Verification items for the finished model (mm, model axes). Coordinates: 2 decimals unless noted, no trailing zeros. Order: outer loops, then holes, each group sorted by start corner. A loop starts at its lowest first (then second) coordinate and runs counter-clockwise, first axis right, second up. Notation, with made-up numbers: M 29.5,30 L 75.5,30 A12 ccw 75.5,48 Z; hole C 40.25,20.5 d1. An arc over 180 degrees is marked long. Answer as a JSON object with one key per item and string values. Group by question number.
(1) Material ranges on line 1 (Z direction, x = -75, y = 0.7); line 2 (Z direction, x = 0, y = 0.7); line 3 (X direction, y = 0.7, z = 76.5), recorded low to high.
(2) Cross-section at C-C (x = 0). Enter the section's corners in (y, z), plus the area to 3 significant figures.
(3) Gauge pin test, flat end, axial feed: pin 1 Ø10 at (x, z) = (-6, 4.5) entering from -Y. Record the tip position at first contact, or that the pin passes through.
(4) Cross-section at D-D (z = -75). Enter the section's corners in (x, y).
(5) Cross-section at A-A (z = 0). Enter the section's corners in (x, y).
(6) Cross-section at B-B (x = 75). Enter the section's corners in (y, z), plus the area to 3 significant figures.
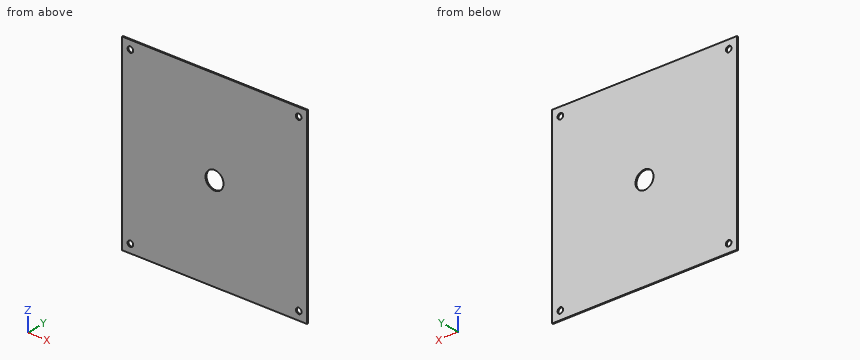
Solid Edge part; units mm, degrees
sketch "Sketch1" plane through (0, 0, 0) normal (0, -1, 0) x (1, 0, 0)
  line L0 (-82.5, -82.5) -> (82.5, -82.5)
  line L1 (82.5, -82.5) -> (82.5, 82.5)
  line L2 (82.5, 82.5) -> (-82.5, 82.5)
  line L3 (-82.5, 82.5) -> (-82.5, -82.5)
  circle A0 centre (0, 0) radius 2
extrude "Protrusion1" add sketch "Sketch1" against normal blind 1
sketch "Sketch2" plane through (0, 0, 0) normal (0, -1, 0) x (1, 0, 0)
  circle A0 centre (0, 0) radius 8
extrude "Cutout1" cut sketch "Sketch2" against normal through all
sketch "Sketch3" plane through (0, 0, 0) normal (0, -1, 0) x (1, 0, 0)
  circle A0 centre (-75, 75) radius 2.5
  circle A1 centre (75, 75) radius 2.5
  circle A2 centre (75, -75) radius 2.5
  circle A3 centre (-75, -75) radius 2.5
extrude "Cutout2" cut sketch "Sketch3" against normal through all
properties material "Aluminum, 1060"
Taken from the geometry:
{
 "1": {"line 1": "z = -82.5 to -77.5, -72.5 to 72.5, 77.5 to 82.5", "line 2": "z = -82.5 to -8, 8 to 82.5", "line 3": "x = -82.5 to -77, -73 to 73, 77 to 82.5"},
 "2": {"outline": "M 0,-82.5 L 1,-82.5 L 1,-8 L 0,-8 Z; M 0,8 L 1,8 L 1,82.5 L 0,82.5 Z", "area": "149 mm²"},
 "3": {"pin 1": "stops at y = 0"},
 "4": {"outline": "M -82.5,0 L -77.5,0 L -77.5,1 L -82.5,1 Z; M -72.5,0 L 72.5,0 L 72.5,1 L -72.5,1 Z; M 77.5,0 L 82.5,0 L 82.5,1 L 77.5,1 Z"},
 "5": {"outline": "M -82.5,0 L -8,0 L -8,1 L -82.5,1 Z; M 8,0 L 82.5,0 L 82.5,1 L 8,1 Z"},
 "6": {"outline": "M 0,-82.5 L 1,-82.5 L 1,-77.5 L 0,-77.5 Z; M 0,-72.5 L 1,-72.5 L 1,72.5 L 0,72.5 Z; M 0,77.5 L 1,77.5 L 1,82.5 L 0,82.5 Z", "area": "155 mm²"}
}
